Geometry check sheet. Reference: the model listing, model coordinates, mm. Face numbers are marked on the shaded views. A direction names the side the tool comes from. Coordinates: 2 decimals unless noted, no trailing zeros. Order: outer loops, then holes, each group sorted by start corner. A loop starts at its lowest first (then second) coordinate and runs counter-clockwise, first axis right, second up. Notation, with made-up numbers: (55, 64) - (90, 64) arc R28 cw to (90, 101) - close; hole circle Ø11 at (6.25, 25). An arc over 180 degrees is marked (long way). Put each result on its own line as item: value.
from build123d import *

# Parameters (mm, degrees)
F1_DEPTH = 1.6256
F3_DEPTH = 2.3876
F5_R     = 12.7
F6_DEPTH = 1.524


with BuildPart() as f1:
    # F0 (on Top) → F1 (new body)
    with BuildSketch(Plane.XY):
        Polygon((-22.8219, -39.52869), (22.8219, -39.52869), (45.6438, 0), (22.8219, 39.52869), (-22.8219, 39.52869), (-45.6438, 0), align=None)
    extrude(amount=F1_DEPTH)

    # F2 (on Top) → F3 (join)
    with BuildSketch(Plane.XY):
        Polygon((-20.006278, -34.65189), (20.006278, -34.65189), (40.012556, 0), (20.006278, 34.65189), (-20.006278, 34.65189), (-40.012556, 0), align=None)
    extrude(amount=F3_DEPTH)

    # F5 (on face) → F6 (cut)
    with BuildSketch(Plane.XY.offset(2.3876)):
        with Locations((22.8219, -39.52869)):
            Circle(F5_R)
        with Locations((45.6438, 0)):
            Circle(F5_R)
        with Locations((22.8219, 39.52869)):
            Circle(F5_R)
        with Locations((-22.8219, 39.52869)):
            Circle(F5_R)
        with Locations((-45.6438, 0)):
            Circle(F5_R)
        with Locations((-22.8219, -39.52869)):
            Circle(F5_R)
    extrude(amount=-F6_DEPTH, mode=Mode.SUBTRACT)


solid = f1.part
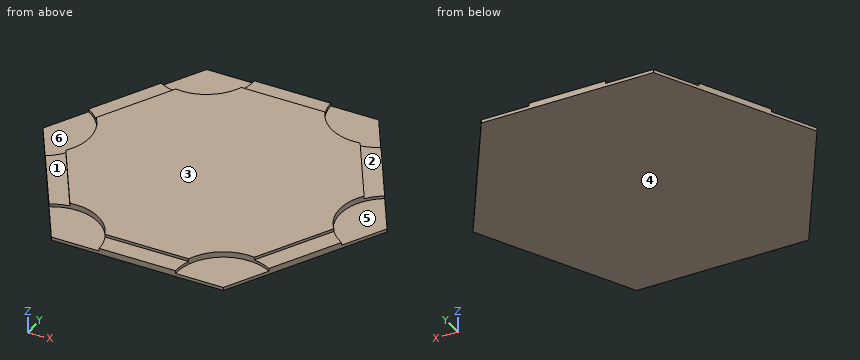
Q1. Section check A-A on x = 2. Record the boundary of the cut face in (y, z).
Answer block:
outline: (-39.53, 0) - (39.53, 0) - (39.53, 1.63) - (34.65, 1.63) - (34.65, 2.39) - (-34.65, 2.39) - (-34.65, 1.63) - (-39.53, 1.63) - close
Q2. Section check D-D on x = -27. Record the boundary of the cut face in (y, z), then the cut area to 3 significant figures.
Answer block:
outline: (-32.29, 0) - (32.29, 0) - (32.29, 0.86) - (27.54, 0.86) - (27.54, 1.63) - (22.54, 1.63) - (22.54, 2.39) - (-22.54, 2.39) - (-22.54, 1.63) - (-27.54, 1.63) - (-27.54, 0.86) - (-32.29, 0.86) - close
area: 132 mm^2
Q3. Draft check along Y on the marked faces 4, 5 and 6. Enter one of: pulls with the +Y half, pulls with the -Y half, needs draft (parallel to the pull), parting line crosses it, or undercut.
Answer block:
face 4: needs draft
face 5: undercut
face 6: undercut
Q4. Depth check by flat-ended pin: pin 1 Ø10 at (x, y) = (20, 33) entering from +Z; pin 2 Ø1 at (y, z) = (-27, 0.5) entering from +X; pin 3 Ø1.5 at (x, y) = (2.5, 37) entering from +Z. Enter the tip coordinate at first touch or a pass-through.
Answer block:
pin 1: stops at z = 0.86
pin 2: stops at x = 30.34
pin 3: stops at z = 1.63
Q5. Section check B-B on z = 0.45. Record the boundary of the cut face in (x, y).
Answer block:
outline: (-45.64, 0) - (-22.82, -39.53) - (22.82, -39.53) - (45.64, 0) - (22.82, 39.53) - (-22.82, 39.53) - close
Q6. Access from +Z, -Z, +X, -X, +Y, -Y to the whole of each face (thin tool, end or side, straight path). Record for the marked faces 1, 2 and 3.
Answer block:
face 1: +Z, -X, -Y
face 2: +Z, +X, +Y
face 3: +Z, +X, -X, +Y, -Y
Q7. Thickness scan on L1, parallel to Z at x = -12.5, y = 34; L2, parallel to Z at x = 36, y = -16.5; L3, parallel to X at y = 19, z = 0.45. Record the ranges inside material, lowest first. Write a range as [from, to].
Answer block:
L1: z = [0, 0.86]
L2: z = [0, 1.63]
L3: x = [-34.67, 34.67]
Q8. Section check C-C on y = -16.5. Record the boundary of the cut face in (x, z).
Answer block:
outline: (-36.12, 0) - (36.12, 0) - (36.12, 1.63) - (30.49, 1.63) - (30.49, 2.39) - (-30.49, 2.39) - (-30.49, 1.63) - (-36.12, 1.63) - close
